from build123d import *

# Parameters (mm, degrees)
BOSS_EXTRUDE1_DEPTH   = 19
SKETCH2_R             = 4
M8_HOLE_DEPTH         = 21
M8_HOLE_DEPTH_BACK    = 5
SKETCH3_R             = 2.5
M5_HOLES_DEPTH        = 21
M5_HOLES_DEPTH_BACK   = 5
SKETCH4_W             = 12
SKETCH4_H             = 20
TRIM_DOWN_SIDES_DEPTH = 25
FILLET3_R             = 2


with BuildPart() as part:
    # Sketch1 → Boss-Extrude1 (new body, symmetric)
    with BuildSketch(Plane.XY):
        Polygon((0, 24), (-4, 24), (-4, 4), (-20, 4), (-20, 24), (-24, 24), (-24, 0), (0, 0), align=None)
    extrude(amount=BOSS_EXTRUDE1_DEPTH, both=True)

    # Sketch2 → M8 hole (cut, two sides)
    with BuildSketch(Plane.ZY.offset(4)) as m8_hole_sk:
        with Locations((0, 18)):
            Circle(SKETCH2_R)
    extrude(amount=M8_HOLE_DEPTH, mode=Mode.SUBTRACT)
    extrude(m8_hole_sk.sketch, amount=-M8_HOLE_DEPTH_BACK, mode=Mode.SUBTRACT)

    # Sketch3 → M5 holes (cut, two sides)
    with BuildSketch(Plane(origin=(0, 4, 0), x_dir=(1, 0, 0), z_dir=(0, 1, 0))) as m5_holes_sk:
        with Locations((-19, 14.5)):
            Circle(SKETCH3_R)
        with Locations((-5, 14.5)):
            Circle(SKETCH3_R)
        with Locations((-5, -14.5)):
            Circle(SKETCH3_R)
        with Locations((-19, -14.5)):
            Circle(SKETCH3_R)
    extrude(amount=M5_HOLES_DEPTH, mode=Mode.SUBTRACT)
    extrude(m5_holes_sk.sketch, amount=-M5_HOLES_DEPTH_BACK, mode=Mode.SUBTRACT)

    # Sketch4 → trim down sides (cut, through all)
    with BuildSketch(Plane.ZY.offset(24)):
        with Locations((-13, 14)):
            Rectangle(SKETCH4_W, SKETCH4_H)
        with Locations((13, 14)):
            Rectangle(SKETCH4_W, SKETCH4_H)
    extrude(amount=-TRIM_DOWN_SIDES_DEPTH, mode=Mode.SUBTRACT)

    # Fillet3
    fillet3_edges = [part.edges().sort_by_distance(p)[0] for p in [
        (-2, 4, 7),
        (-22, 4, 7),
        (-20, 4, 0),
        (-4, 4, 0),
        (-22, 4, -7),
        (-2, 4, -7),
    ]]
    fillet(fillet3_edges, radius=FILLET3_R)


solid = part.part
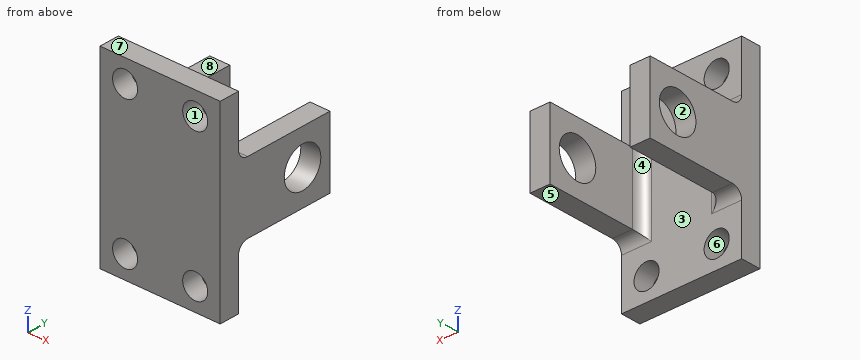
Design review of the part built by this model. Coordinates are the model's own, in mm. Face numbers are marked on the shaded views. A direction names the side the tool comes from. Coordinates: 2 decimals unless noted, no trailing zeros. Loops run counter-clockwise (first coordinate to the right, second up) from the corner with the lowest first, then second, coordinate; pieces in that order, holes last. Notation, with made-up numbers: M 51,-30.75 L 75,-30.75 A14 ccw 75,-23.75 Z; hole C -40,76 d9. An arc over 180 degrees is marked long. Use one line per item in the form item = value.
(1) Draft analysis for pull direction Y (two halves, no side actions). For the marked faces 1, 2 and 3, state which applies: pulls with the +Y half, pulls with the -Y half, needs draft (parallel to the pull), parting line crosses it, or undercut.
Return value:
face_1 = needs draft
face_2 = undercut
face_3 = pulls with the +Y half
(2) Consider section B-B (y = 18). Write out the cut boundary in (x, z).
Return value:
outline = M -24,-7 L -20,-7 L -20,-4 L -24,-4 Z; M -24,4 L -20,4 L -20,7 L -24,7 Z; M -4,-7 L 0,-7 L 0,-4 L -4,-4 Z; M -4,4 L 0,4 L 0,7 L -4,7 Z
(3) Consider section C-C (y = 8.75). Write out the cut boundary in (x, z), and give its area (3 significant figures).
Return value:
outline = M -24,-7 L -20,-7 L -20,7 L -24,7 Z; M -4,-7 L 0,-7 L 0,7 L -4,7 Z
area = 112 mm2
(4) For line 1 along Z through (x, y) = (-19, 1.35); line 2 along X through (y, z) = (1.45, 14.5); line 3 along X through (y, z) = (13.75, -1.5), list the stretches that pass through material, from the lowest coordinate up. Write a range as from..to.
Return value:
line_1 = -19..-17, -12..12, 17..19
line_2 = -24..-21.5, -16.5..-7.5, -2.5..0
line_3 = -24..-20, -4..0
(5) Consider section D-D (x = -19). Write out the cut boundary in (y, z).
Return value:
outline = M 0,-19 L 4,-19 L 4,-17 L 0,-17 Z; M 0,-12 L 4,-12 L 4,-9 A2 cw 4.27,-8 L 4.27,8 A2 cw 4,9 L 4,12 L 0,12 Z; M 0,17 L 4,17 L 4,19 L 0,19 Z
(6) Consider section A-A (z = 0). Write out the cut boundary in (x, y), and give its area (3 significant figures).
Return value:
outline = M -24,0 L 0,0 L 0,14 L -4,14 L -4,6 A2 cw -6,4 L -18,4 A2 cw -20,6 L -20,14 L -24,14 Z; M -24,22 L -20,22 L -20,24 L -24,24 Z; M -4,22 L 0,22 L 0,24 L -4,24 Z
area = 194 mm2
(7) Clearance check with flat-ended pins moving along their axes: P1, Ø1.2, axis at x = -2, y = 16, coming from the -Z side; P2, Ø5, axis at x = -5.5, z = 13.5, coming from the +Y side; P3, Ø3, axis at x = -3, y = 15, coming from the +Z side. State where each tip first meets the part, or that it passes through.
Return value:
P1 = -7
P2 = 4
P3 = 7
(8) For the marked faces 4, 5, 6, 7 and 8, list the 3-axis set-ups (+Z, -Z, +X, -X, +Y, -Y) from which the entire face can be reached by the end or side of a thin tool; tool diameter is ignored.
Return value:
face_4 = +Z, -Z, +Y
face_5 = -Z, +X, -X, +Y
face_6 = +Y, -Y
face_7 = +Z, +X, -X, +Y, -Y
face_8 = +Z, +X, -X, +Y
